Can you work these out from the model? Positions are in its coordinate system, mm. A direction names the side the tool comes from. Give positions to 0.01 mm unless a question says otherwise; leave off trailing zeros. Loops run counter-clockwise (first coordinate to the right, second up) from the corner with the lowest first, then second, coordinate; pieces in that order, holes last. Notation, with made-up numbers: M 54.25,11.5 L 92.25,11.5 A19 cw 92.25,22.5 Z; hole C 27.5,50.5 d11. An arc over 180 degrees is marked long. Answer as a JSON object with one key per item and string values.
```python
from build123d import *

# Parameters (mm, degrees)
SKETCH2_W           = 140
SKETCH2_H           = 200
BOSS_EXTRUDE1_DEPTH = 4
BOSS_EXTRUDE2_DEPTH = 5
SKETCH4_R           = 3
CUT_EXTRUDE1_DEPTH  = 10


with BuildPart() as part:
    # Sketch2 → Boss-Extrude1 (new body)
    with BuildSketch(Plane(origin=(0, 0, 0), x_dir=(1, 0, 0), z_dir=(0, 1, 0))):
        with Locations((70, 100)):
            Rectangle(SKETCH2_W, SKETCH2_H)
    extrude(amount=-BOSS_EXTRUDE1_DEPTH)

    # Sketch1 → Boss-Extrude2 (add)
    with BuildSketch(Plane(origin=(0, 0, 0), x_dir=(1, 0, 0), z_dir=(0, 1, 0))):
        with BuildLine():
            Line((83.253956867, 58.796283012), (118.253956867, 28.796283012))
            ThreePointArc((118.253956867, 28.796283012), (118.796283012, 21.746043133), (111.746043133, 21.203716988))
            Line((111.746043133, 21.203716988), (76.746043133, 51.203716988))
            ThreePointArc((76.746043133, 51.203716988), (76.203716988, 58.253956867), (83.253956867, 58.796283012))
        make_face()
        with BuildLine():
            Line((65, 75), (65, 125))
            ThreePointArc((65, 125), (70, 130), (75, 125))
            Line((75, 125), (75, 75))
            ThreePointArc((75, 75), (70, 70), (65, 75))
        make_face()
        with BuildLine():
            Line((56.746043133, 58.796283012), (21.746043133, 28.796283012))
            ThreePointArc((21.746043133, 28.796283012), (21.203716988, 21.746043133), (28.253956867, 21.203716988))
            Line((28.253956867, 21.203716988), (63.253956867, 51.203716988))
            ThreePointArc((63.253956867, 51.203716988), (63.796283012, 58.253956867), (56.746043133, 58.796283012))
        make_face()
        with BuildLine():
            Line((56.746043133, 141.203716988), (21.746043133, 171.203716988))
            ThreePointArc((21.746043133, 171.203716988), (21.203716988, 178.253956867), (28.253956867, 178.796283012))
            Line((28.253956867, 178.796283012), (63.253956867, 148.796283012))
            ThreePointArc((63.253956867, 148.796283012), (63.796283012, 141.746043133), (56.746043133, 141.203716988))
        make_face()
        with BuildLine():
            Line((83.253956867, 141.203716988), (118.253956867, 171.203716988))
            ThreePointArc((118.253956867, 171.203716988), (118.796283012, 178.253956867), (111.746043133, 178.796283012))
            Line((111.746043133, 178.796283012), (76.746043133, 148.796283012))
            ThreePointArc((76.746043133, 148.796283012), (76.203716988, 141.746043133), (83.253956867, 141.203716988))
        make_face()
    extrude(amount=BOSS_EXTRUDE2_DEPTH)

    # Sketch4 → Cut-Extrude1 (cut)
    with BuildSketch(Plane(origin=(0, 0, 0), x_dir=(1, 0, 0), z_dir=(0, 1, 0))):
        with Locations(Location((70, 191.8, 0), (0, 0, 270))):
            Circle(SKETCH4_R)
        with Locations(Location((8.166074554, 133, 0), (0, 0, 270))):
            Circle(SKETCH4_R)
        with Locations(Location((70, 8.2, 0), (0, 0, 90))):
            Circle(SKETCH4_R)
        with Locations(Location((8.166074554, 67, 0), (0, 0, 90))):
            Circle(SKETCH4_R)
        with Locations(Location((131.833925446, 67, 0), (0, 0, 270))):
            Circle(SKETCH4_R)
        with Locations(Location((131.833925446, 133, 0), (0, 0, 90))):
            Circle(SKETCH4_R)
    extrude(amount=-CUT_EXTRUDE1_DEPTH, mode=Mode.SUBTRACT)


solid = part.part
```
1) Suppose I cut it at B-B, the plane x = 70. Write out the boundary of the cut face in (y, z).
Answer list:
{"outline": "M -4,-200 L 0,-200 L 0,-194.8 L -4,-194.8 Z; M -4,-188.8 L 0,-188.8 L 0,-130 L 5,-130 L 5,-70 L 0,-70 L 0,-11.2 L -4,-11.2 Z; M -4,-5.2 L 0,-5.2 L 0,0 L -4,0 Z"}
2) Suppose I cut it at C-C, the plane z = -8.2. Write out the boundary of the cut face in (x, y).
Answer list:
{"outline": "M 0,-4 L 67,-4 L 67,0 L 0,0 Z; M 73,-4 L 140,-4 L 140,0 L 73,0 Z"}
3) Will these pins go through, and if not, where does the flat tip stop? pin 1 Ø9.5 at (x, z) = (8.17, -133) entering from -Y; pin 2 Ø2 at (y, z) = (2.5, -86.5) entering from -X; pin 3 Ø9.5 at (x, z) = (70, -191.8) entering from +Y.
Answer list:
{"pin 1": "y = -4", "pin 2": "x = 65", "pin 3": "y = 0"}
4) Suppose I cut it at D-D, the plane z = -91. Write out the boundary of the cut face in (x, y).
Answer list:
{"outline": "M 0,-4 L 140,-4 L 140,0 L 75,0 L 75,5 L 65,5 L 65,0 L 0,0 Z"}
5) If we mould it in two halves opening along X, with no side actions, what happens to faces 1 (the flat face through (100.509, 2.465, -155.994)), 2 (the cylindrical face through (9.99, -1.97, -64.62)), 3 (the cylindrical face through (134.81, -1.97, -67.39)), 4 (the flat face through (42, 5, -42))? For each: +X half, -X half, draft (parallel to the pull), parting line (faces both ways), or undercut.
Answer list:
{"face 1": "+X half", "face 2": "undercut", "face 3": "undercut", "face 4": "draft"}
6) For faces 5 (the flat face through (94.491, 2.465, -164.006)), 6 (the cylindrical face through (64, 2, -142)), 7 (the flat face through (75, 2, -100)), which set-ups out of +Z, -Z, +X, -X, +Y, -Y let a thin tool reach every point of the face, with its end or its side?
Answer list:
{"face 5": "-Z, +Y", "face 6": "+Y", "face 7": "+X, +Y"}
7) Please list where these lines run through material, in increasing order: line 1 along X through (y, z) = (-2.6, -67); line 2 along X through (y, z) = (-3.1, -191.8); line 3 along Y through (x, z) = (74, -172.5). Write a range as from..to.
Answer list:
{"line 1": "0..5.17, 11.17..128.83, 134.83..140", "line 2": "0..67, 73..140", "line 3": "-4..0"}
8) Suppose I cut it at A-A, the plane y = 3.5. Write out the boundary of the cut face in (x, z), and give its area (3 significant figures).
Answer list:
{"outline": "M 21.75,-171.2 A5 ccw 28.25,-178.8 L 63.25,-148.8 A5 ccw 56.75,-141.2 Z; M 21.75,-28.8 L 56.75,-58.8 A5 ccw 63.25,-51.2 L 28.25,-21.2 A5 ccw Z; M 65,-125 A5 ccw 75,-125 L 75,-75 A5 ccw 65,-75 Z; M 76.75,-148.8 L 111.75,-178.8 A5 ccw 118.25,-171.2 L 83.25,-141.2 A5 ccw Z; M 76.75,-51.2 A5 ccw 83.25,-58.8 L 118.25,-28.8 A5 ccw 111.75,-21.2 Z", "area": "2,740 mm^2"}
